from build123d import *

# Parameters (mm, degrees)
AUFSATZ_LINEAR_AUSTRAGEN1_DEPTH = 100
SKIZZE4_R                       = 4.5
AUFSATZ_LINEAR_AUSTRAGEN2_DEPTH = 15
VERRUNDUNG1_R                   = 10


with BuildPart() as part:
    # Skizze1 → Aufsatz-Linear austragen1 (new body)
    with BuildSketch(Plane.XY):
        Polygon((-5.5, 0), (-5.5, 30), (-4, 30), (0, 7.314872722), (4, 7.314872722), (8, 30), (9.5, 30), (9.5, 0), align=None)
    extrude(amount=AUFSATZ_LINEAR_AUSTRAGEN1_DEPTH)

    # Skizze4 → Aufsatz-Linear austragen2 (add)
    with BuildSketch(Plane.ZY.offset(5.5)):
        with BuildLine():
            Line((100, 30), (145, 30))
            Line((145, 30), (145, -25))
            Line((145, -25), (104.142135624, -25))
            ThreePointArc((104.142135624, -25), (100.3153013, -24.238795325), (97.071067812, -22.071067812))
            Line((97.071067812, -22.071067812), (75, 0))
            Line((75, 0), (100, 0))
            Line((100, 0), (100, 30))
        make_face()
        with Locations((122.5, 20)):
            Circle(SKIZZE4_R, mode=Mode.SUBTRACT)
        with Locations((122.5, -15)):
            Circle(SKIZZE4_R, mode=Mode.SUBTRACT)
    extrude(amount=-AUFSATZ_LINEAR_AUSTRAGEN2_DEPTH)

    # Verrundung1
    verrundung1_edges = [part.edges().sort_by_distance(p)[0] for p in [
        (2, 0, 75),
    ]]
    fillet(verrundung1_edges, radius=VERRUNDUNG1_R)


solid = part.part
Can you work these out from the model? Positions are in its coordinate system, mm. A direction names the side the tool comes from. Coordinates: 2 decimals unless noted, no trailing zeros. Write each loop counter-clockwise with the first axis right and the second up, starting at its lowest first coordinate (ties: lowest second). Pieces come first, ordered by that corner, then holes.
Q1. If we mould it in two halves opening along Y, with no side actions, what happens to faces 4 (the face through (2.11, -0.74, 74.63)), 5 (the face through (2, 20, 118)), 6 (the face through (-2.03, 18.82, 49.3)), 7 (the face through (2, 3, 145))? For each: +Y half, -Y half, draft (parallel to the pull), parting line (faces both ways), or undercut.
Results found:
face 4: -Y half
face 5: undercut
face 6: +Y half
face 7: draft
Q2. For P1, Ø6, axis at x = 7.5, z = 70.5, coming from the -Y side; P2, Ø4.5, axis at x = 0, z = 35.5, coming from the -Y side; P3, Ø6, axis at x = 5.5, y = -5, coming from the -Z side, each with a flat end and sliding along its axis, tell me the tip position at first contact or that it passes through.
Results found:
P1: stops at y = -0.36
P2: stops at y = 0
P3: stops at z = 76.86
Q3. Imagine slicing it at C-C, the plane y = -15. List the corners of the cut face in (x, z) for me.
Results found:
outline: (-5.5, 90) - (9.5, 90) - (9.5, 118) - (-5.5, 118) - close; (-5.5, 127) - (9.5, 127) - (9.5, 145) - (-5.5, 145) - close
Q4. Which directions (+Z, -Z, +X, -X, +Y, -Y) give clear straight access to the entire face, cutting with the end or side of a thin tool? Please do faces 1 (the face through (2, 0, 35)), 2 (the face through (2, 7.315, 49)), 3 (the face through (5, 12, 0)).
Results found:
face 1: -Z, +X, -X, -Y
face 2: -Z, +Y
face 3: -Z, +X, -X, +Y, -Y
Q5. Imagine slicing it at D-D, the plane z = 58. List the corners of the cut face in (x, y) for me, plus the area to 3 significant figures.
Results found:
outline: (-5.5, 0) - (9.5, 0) - (9.5, 30) - (8, 30) - (4, 7.31) - (0, 7.31) - (-4, 30) - (-5.5, 30) - close
area: 269 mm2
Q6. Imagine slicing it at A-A, the plane z = 122.5. List the corners of the cut face in (x, y) for me, plus the area to 3 significant figures.
Results found:
outline: (-5.5, -25) - (9.5, -25) - (9.5, -19.5) - (-5.5, -19.5) - close; (-5.5, -10.5) - (9.5, -10.5) - (9.5, 15.5) - (-5.5, 15.5) - close; (-5.5, 24.5) - (9.5, 24.5) - (9.5, 30) - (-5.5, 30) - close
area: 555 mm2
Q7. Please list where these lines run through material, in increasing order: L1, parallel to Y at x = -1.25, z = 122.5; L2, parallel to Z at x = -1.25, y = -13.5; L3, parallel to X at y = 9, z = 76.5.
Results found:
L1: y = -25 to -19.5, -10.5 to 15.5, 24.5 to 30
L2: z = 88.5 to 118.26, 126.74 to 145
L3: x = -5.5 to -0.3, 4.3 to 9.5
Q8. Imagine slicing it at B-B, the plane x = 1.25. List the corners of the cut face in (y, z) for me.
Results found:
outline: (-25, 104.14) arc R10 ccw to (-22.07, 97.07) - (-2.93, 77.93) arc R10 cw to (0, 70.86) - (0, 0) - (7.31, 0) - (7.31, 100) - (30, 100) - (30, 145) - (-25, 145) - close; hole circle Ø9 at (-15, 122.5); hole circle Ø9 at (20, 122.5)
